For this review, take the finished solid that the model builds, in its own axes (mm). Face numbers are marked on the shaded views. A direction names the side the tool comes from. Give positions to 0.01 mm unless a question says otherwise; leave off trailing zeros. Write each loop counter-clockwise with the first axis right and the second up, starting at its lowest first coordinate (ties: lowest second). Pieces come first, ordered by that corner, then holes. Notation, with made-up numbers: (80, -3) -> (93, -3) arc R21 ccw to (93, 6) -> close; hole circle Ø11 at (76, 57.25). An arc over 180 degrees is marked (long way). Write item = value, one per line.
```python
from build123d import *

# Parameters (mm, degrees)
SKETCH1_W           = 18
SKETCH1_H           = 27
SKETCH1_R           = 4.5
SKETCH1_W_2         = 42
SKETCH1_H_2         = 6
BOSS_EXTRUDE1_DEPTH = 14
SKETCH2_R           = 2.25
CUT_EXTRUDE1_DEPTH  = 37.959437225
CUT_EXTRUDE2_DEPTH  = 40.204591568
CUT_EXTRUDE3_REACH  = 46.677
SKETCH4_R           = 2.25


with BuildPart() as part:
    # Sketch1 → Boss-Extrude1 (new body)
    # profile 1 of 2: a face of its own
    with BuildSketch(Plane.XY):
        with Locations((0, 16.5)):
            Rectangle(SKETCH1_W, SKETCH1_H)
        with Locations((0, 17)):
            Circle(SKETCH1_R, mode=Mode.SUBTRACT)
    # profile 2 of 2: a face of its own
    with BuildSketch(Plane.XY):
        Rectangle(SKETCH1_W_2, SKETCH1_H_2)
    extrude(amount=BOSS_EXTRUDE1_DEPTH)

    # Sketch2 → Cut-Extrude1 (cut, through all)
    with BuildSketch(Plane(origin=(0, 3, 0), x_dir=(1, 0, 0), z_dir=(0, 1, 0))):
        with Locations(Location((-16, -7, 0), (0, 0, 270))):
            Circle(SKETCH2_R)
        with Locations(Location((16, -7, 0), (0, 0, 90))):
            Circle(SKETCH2_R)
    extrude(amount=-CUT_EXTRUDE1_DEPTH, mode=Mode.SUBTRACT)

    # Sketch3 → Cut-Extrude2 (cut, through all)
    with BuildSketch(Plane.XY.offset(14)):
        with BuildLine():
            Line((0.5, 30), (0.5, 21.472135955))
            ThreePointArc((0.5, 21.472135955), (0, 21.5), (-0.5, 21.472135955))
            Line((-0.5, 21.472135955), (-0.5, 30))
            Line((-0.5, 30), (0.5, 30))
        make_face()
    extrude(amount=-CUT_EXTRUDE2_DEPTH, mode=Mode.SUBTRACT)

    # Cut-Extrude3: up to this face of the body (flat: up to its plane)
    cut_extrude3_end = Plane(part.part.faces().sort_by_distance((-9, 16.5, 7))[0])
    # Sketch4 → Cut-Extrude3 (cut, up to the picked face)
    with BuildSketch(Plane(origin=(9, 0, 0), x_dir=(0, 0, -1), z_dir=(1, 0, 0)), mode=Mode.PRIVATE) as cut_extrude3_sk1:
        with Locations((-6.695292014, 25.95)):
            Circle(SKETCH4_R)
    cut_extrude3_tool1 = split(extrude(cut_extrude3_sk1.sketch, amount=-CUT_EXTRUDE3_REACH, mode=Mode.PRIVATE), bisect_by=cut_extrude3_end, keep=Keep.BOTH, mode=Mode.PRIVATE)
    add(cut_extrude3_tool1.solids().sort_by(Axis((9, 25.95, 6.695292), (-1, 0, 0)))[0], mode=Mode.SUBTRACT)


solid = part.part
```
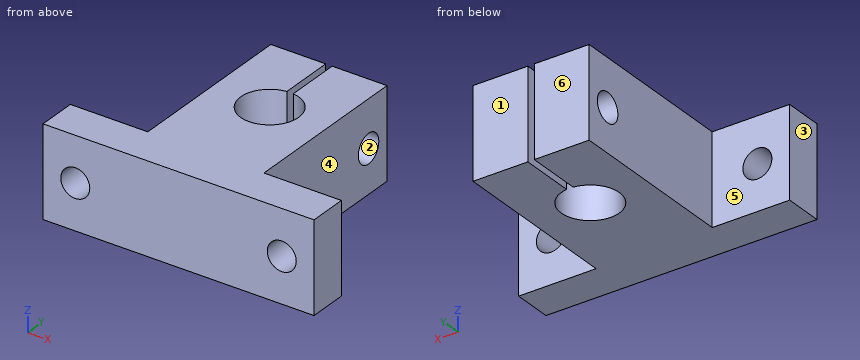
(1) To check wall thickness, follow probe 1 along X at (y, z) = (-0.4, 7); probe 2 along Z at (x, y) = (16, 1); probe 3 along X at (y, z) = (24.5, 1.5). State the ranges of each line that lie inside material, in increasing order.
Answers below:
probe_1 = -21 to -18.25, -13.75 to 13.75, 18.25 to 21
probe_2 = 0 to 4.75, 9.25 to 14
probe_3 = -9 to -0.5, 0.5 to 9
(2) Tool access review of the marked faces 4, 5 and 6: name each direction out of +Z, -Z, +X, -X, +Y, -Y from which nothing blocks a thin tool from reaching the whole face with its end or side.
Answers below:
face_4 = +Z, -Z, +X, +Y
face_5 = +Z, -Z, -X, +Y
face_6 = +Z, -Z, +X, -X, +Y
(3) For pin 1 (3.5 mm diameter, centred on x = 14.5, z = 5.5, fed in from +Y); pin 2 (3.5 mm diameter, centred on y = 25.95, z = 6.7, fed in from -X); pin 3 (6 mm diameter, centred on x = -16, z = 7, fed in from -Y); pin 4 (7 mm diameter, centred on y = 25.95, z = 6.7, fed in from +X), all flat-tipped, find the tip position at first contact; note any pin that passes through.
Answers below:
pin_1 = 3
pin_2 = through
pin_3 = -3
pin_4 = 9
(4) Take a section at D-D (z = 7). Write out the cut boundary in (x, y).
Answers below:
outline = (-21, -3) -> (-18.25, -3) -> (-18.25, 3) -> (-21, 3) -> close; (-13.75, -3) -> (13.75, -3) -> (13.75, 3) -> (9, 3) -> (9, 23.72) -> (0.5, 23.72) -> (0.5, 21.47) arc R4.5 cw (long way) to (-0.5, 21.47) -> (-0.5, 23.72) -> (-9, 23.72) -> (-9, 3) -> (-13.75, 3) -> close; (-9, 28.18) -> (-0.5, 28.18) -> (-0.5, 30) -> (-9, 30) -> close; (0.5, 28.18) -> (9, 28.18) -> (9, 30) -> (0.5, 30) -> close; (18.25, -3) -> (21, -3) -> (21, 3) -> (18.25, 3) -> close
(5) Take a section at A-A (y = 25.95). Write out the cut boundary in (x, z).
Answers below:
outline = (-9, 0) -> (-0.5, 0) -> (-0.5, 4.45) -> (-9, 4.45) -> close; (-9, 8.95) -> (-0.5, 8.95) -> (-0.5, 14) -> (-9, 14) -> close; (0.5, 0) -> (9, 0) -> (9, 4.45) -> (0.5, 4.45) -> close; (0.5, 8.95) -> (9, 8.95) -> (9, 14) -> (0.5, 14) -> close
(6) Take a section at B-B (x = -16). Write out the cut boundary in (y, z), plus the area to 3 significant figures.
Answers below:
outline = (-3, 0) -> (3, 0) -> (3, 4.75) -> (-3, 4.75) -> close; (-3, 9.25) -> (3, 9.25) -> (3, 14) -> (-3, 14) -> close
area = 57.0 mm^2
(7) Take a section at C-C (y = 17). Write out the cut boundary in (x, z), plus the area to 3 significant figures.
Answers below:
outline = (-9, 0) -> (-4.5, 0) -> (-4.5, 14) -> (-9, 14) -> close; (4.5, 0) -> (9, 0) -> (9, 14) -> (4.5, 14) -> close
area = 126 mm^2
(8) The part is to be moulded in two halves that separate along Y. For the marked faces 1, 2 and 3, say which applies: released by +Y, released by -Y, zero draft, split by the parting line, or undercut.
Answers below:
face_1 = released by +Y
face_2 = undercut
face_3 = zero draft
